Input: part model. Units: mm. Frame: model coordinates. A direction names the side the tool comes from. Coordinates: 2 decimals unless noted, no trailing zeros. Write each loop counter-clockwise with the first axis right and the second up, starting at its lowest first coordinate (ties: lowest second). Pieces come first, ordered by that corner, then holes. Notation, with made-up numbers: (15.25, 62) - (31.25, 62) arc R10 cw to (31.25, 77) - close; hole circle Ø1 at (12.5, 15.25). An arc over 180 degrees is marked (long way). One line per question, with ' | ' between items. Start each with the question number.
1) Section query C-C on y = -55.5. Return loops of the section in (x, z), and give its area (3 significant figures).
2) Line query: line 1 (Z direction, x = 0, y = -62); line 2 (Z direction, x = 0, y = -10.9); line 3 (X direction, y = -10.5, z = -3.5). Output: solid intervals per line, ascending.
3) Section query A-A on x = 0. Return loops of the section in (y, z), and give its area (3 significant figures).
4) Section query B-B on z = 0. Return loops of the section in (x, y).
5) Reachability of faces 5 (the flat face through (-11, 0, 17)), 6 (the flat face through (19, -128.4, -8)) from +Z, -Z, +X, -X, +Y, -Y: full face, straight path, thin tool, end or side. Return the list, or none.
6) Draft query along X for faces 1 (the cylindrical face through (23.846, -70.98, 7.509)), 2 (the cylindrical face through (-4.336, -135.07, -19.524)), 3 (the cylindrical face through (-4.336, -5.07, -19.524)), 4 (the flat face through (-11, -140, 17)). Return one class per face: released by +X, released by -X, zero draft, split by the parting line, or undercut.
7) First-contact query: P1, Ø1, axis at x = -3.5, y = -72.5, coming from the +Z side; P2, Ø6, axis at x = 13.5, y = -99, coming from the -Z side; P3, Ø25, axis at x = 0, z = 0, coming from the -Y side; P4, Ø4, axis at x = -7.5, y = -106.5, coming from the -Z side. Flat tips, straight axial feed; report the tip coordinate or a pass-through.
Autodesk Inventor part; units mm, degrees
ref_plane "YZ Plane" through (0, 0, 0) normal (1, 0, 0) x (0, 1, 0)
ref_plane "XZ Plane" through (0, 0, 0) normal (0, 1, 0) x (-1, 0, 0)
ref_plane "XY Plane" through (0, 0, 0) normal (0, 0, 1) x (1, 0, 0)
sketch "Эскиз1" plane through (0, 0, 0) normal (0, 0, 1) x (1, 0, 0)
  line L0 (0, 0) -> (0, -140)
  line L1 (0, 0) -> (20, 0) construction
  line L2 (25, 0) -> (25, -140)
  line L3 (25, -140) -> (20, -140)
  line L4 (20, 0) -> (20, -10)
  line L5 (20, -10) -> (21, -10)
  line L6 (21, -10) -> (21, -11.6)
  line L7 (21, -11.6) -> (20, -11.6)
  line L8 (20, -11.6) -> (20, -128.4)
  line L9 (20, -128.4) -> (21, -128.4)
  line L10 (21, -128.4) -> (21, -130)
  line L11 (21, -130) -> (20, -130)
  line L12 (20, -130) -> (20, -140)
  line L13 (20, -140) -> (0, -140) construction
  line L14 (20, 0) -> (25, 0)
  point P0 (20, -7)
  dimension "d0" = 140
  dimension "d1" = 50
  dimension "d3" = 42
  dimension "d4" = 40
  dimension "d5" = 1.6
  dimension "d6" = 1.6
  dimension "d13" = 10
  dimension "d14" = 10
revolve "Вращение1" add sketch "Эскиз1" angle 360 about axis through (0, 0, 0) along (0, -1, 0)
equation "\"d14\" = my_parameter"
equation "\"my_parameter\" = 10"
properties part number "корпус"
Answer key:
1) outline: circle Ø50 at (0, 0); hole circle Ø40 at (0, 0) | area: 707 mm²
2) line 1: -25 to -20, 20 to 25 | line 2: -25 to -21, 21 to 25 | line 3: -24.75 to -20.71, 20.71 to 24.75
3) outline: (-140, -25) - (0, -25) - (0, -20) - (-10, -20) - (-10, -21) - (-11.6, -21) - (-11.6, -20) - (-128.4, -20) - (-128.4, -21) - (-130, -21) - (-130, -20) - (-140, -20) - close; (-140, 20) - (-130, 20) - (-130, 21) - (-128.4, 21) - (-128.4, 20) - (-11.6, 20) - (-11.6, 21) - (-10, 21) - (-10, 20) - (0, 20) - (0, 25) - (-140, 25) - close | area: 1,390 mm²
4) outline: (-25, -140) - (-20, -140) - (-20, -130) - (-21, -130) - (-21, -128.4) - (-20, -128.4) - (-20, -11.6) - (-21, -11.6) - (-21, -10) - (-20, -10) - (-20, 0) - (-25, 0) - close; (20, -140) - (25, -140) - (25, 0) - (20, 0) - (20, -10) - (21, -10) - (21, -11.6) - (20, -11.6) - (20, -128.4) - (21, -128.4) - (21, -130) - (20, -130) - close
5) face 5: +Z, -Z, +X, -X, +Y | face 6: none
6) face 1: split by the parting line | face 2: undercut | face 3: undercut | face 4: zero draft
7) P1: z = 24.82 | P2: z = -22.69 | P3: through | P4: z = -24.39
